from build123d import *

# Parameters (mm, degrees)
SKETCH1_W           = 60
SKETCH1_H           = 50
BOSS_EXTRUDE3_DEPTH = 3
SKETCH3_R           = 10
SKETCH3_R_2         = 5
CUT_EXTRUDE1_DEPTH  = 889.569461306
SKETCH4_R           = 2.5
CUT_EXTRUDE2_DEPTH  = 10


with BuildPart() as part:
    # Sketch1 → Boss-Extrude3 (new body)
    with BuildSketch(Plane.XY):
        Polygon((-630, 258.933751306), (-790, 138.933751306), (-790, 88.933751306), (-630, 208.933751306), (-530, 208.933751306), (-60, -25), (60, -25), (60, 25), (-60, 25), (-530, 258.933751306), align=None)
        with Locations((-820, 113.933751306)):
            Rectangle(SKETCH1_W, SKETCH1_H)
    extrude(amount=BOSS_EXTRUDE3_DEPTH)

    # Sketch3 → Cut-Extrude1 (cut, through all)
    with BuildSketch(Plane.XY.offset(3)):
        with Locations((-580, 233.933751306)):
            Circle(SKETCH3_R)
        with Locations((-820, 113.933751306)):
            Circle(SKETCH3_R)
        with Locations((40, -15)):
            Circle(SKETCH3_R_2)
        with Locations((-40, -15)):
            Circle(SKETCH3_R_2)
    extrude(amount=-CUT_EXTRUDE1_DEPTH, mode=Mode.SUBTRACT)

    # Sketch4 → Cut-Extrude2 (cut)
    with BuildSketch(Plane.XY.offset(3)):
        with Locations((-548, 233.933751306)):
            Circle(SKETCH4_R)
        with Locations((-612, 233.933751306)):
            Circle(SKETCH4_R)
    extrude(amount=-CUT_EXTRUDE2_DEPTH, mode=Mode.SUBTRACT)


solid = part.part
The model under review builds one solid part; all positions refer to its coordinate system, in mm. A direction names the side the tool comes from. Round coordinates to 2 decimals unless told otherwise and drop trailing zeros. Order: outer loops, then holes, each group sorted by start corner. A loop starts at its lowest first (then second) coordinate and runs counter-clockwise, first axis right, second up. Notation, with made-up numbers: (64.25, 70) -> (115.25, 70) arc R29 cw to (115.25, 104) -> close; hole circle Ø2 at (20.25, 28). An arc over 180 degrees is marked (long way). Write item = value, one per line. Start each with the question number.
Item 1: Clearance check with flat-ended pins moving along their axes: pin 1 Ø8 at (x, y) = (40, -15) entering from +Z; pin 2 Ø1 at (y, z) = (73, 2.5) entering from -X; pin 3 Ø1.5 at (x, z) = (-510.5, 0.5) entering from -Y; pin 4 Ø0.9 at (x, z) = (-827.5, 1.5) entering from -Y. State where each tip first meets the part, or that it passes through.
Item 2: Consider section C-C on z = 1.4. Write out the cut boundary in (x, y).
Item 3: Consider section B-B on y = 192.5. Write out the cut boundary in (x, z), plus the area to 3 significant figures.
Item 4: For line 1 along X through (y, z) = (105.5, 0.6); line 2 along Y through (x, z) = (-612, 0.85); line 3 along Y through (x, z) = (40, 0.75), list the stretches that pass through material, from the lowest coordinate up.
Item 5: Mouldability with a two-part tool opening along X and no side actions: class faces 1 (the face through (-708.88, 199.774, 1.479)), 2 (the face through (-397, 160, 3)), 3 (the face through (-711.12, 148.094, 1.479)) as released by +X, released by -X, zero draft, split by the parting line, or undercut.
Item 6: For faces 4 (the face through (-291.71, 140.33, 1.48)), 5 (the face through (-298.29, 93.604, 1.479)), list the 3-axis set-ups (+Z, -Z, +X, -X, +Y, -Y) from which the entire face can be reached by the end or side of a thin tool; tool diameter is ignored.
Item 7: Consider section D-D on y = 80.5. Write out the cut boundary in (x, z), plus the area to 3 significant figures.
Item 8: Consider section A-A on x = -820. Write out the cut boundary in (y, z), plus the area to 3 significant figures.
Conclusion:
q1.pin_1 = through
q1.pin_2 = -257.9
q1.pin_3 = 198.85
q1.pin_4 = 88.93
q2.outline = (-850, 88.93) -> (-790, 88.93) -> (-630, 208.93) -> (-530, 208.93) -> (-60, -25) -> (60, -25) -> (60, 25) -> (-60, 25) -> (-530, 258.93) -> (-630, 258.93) -> (-790, 138.93) -> (-850, 138.93) -> close; hole circle Ø20 at (-820, 113.93); hole circle Ø5 at (-612, 233.93); hole circle Ø20 at (-580, 233.93); hole circle Ø5 at (-548, 233.93); hole circle Ø10 at (-40, -15); hole circle Ø10 at (40, -15)
q3.outline = (-718.58, 0) -> (-651.91, 0) -> (-651.91, 3) -> (-718.58, 3) -> close; (-496.98, 0) -> (-396.53, 0) -> (-396.53, 3) -> (-496.98, 3) -> close
q3.area = 501 mm2
q4.line_1 = -850 to -825.37, -814.63 to -767.91, -322.19 to -221.73
q4.line_2 = 208.93 to 231.43, 236.43 to 258.93
q4.line_3 = -25 to -20, -10 to 25
q5.face_1 = released by -X
q5.face_2 = zero draft
q5.face_3 = undercut
q6.face_4 = +Z, -Z, +X, +Y
q6.face_5 = +Z, -Z, -Y
q7.outline = (-271.96, 0) -> (-171.51, 0) -> (-171.51, 3) -> (-271.96, 3) -> close
q7.area = 301 mm2
q8.outline = (88.93, 0) -> (103.93, 0) -> (103.93, 3) -> (88.93, 3) -> close; (123.93, 0) -> (138.93, 0) -> (138.93, 3) -> (123.93, 3) -> close
q8.area = 90.0 mm2
